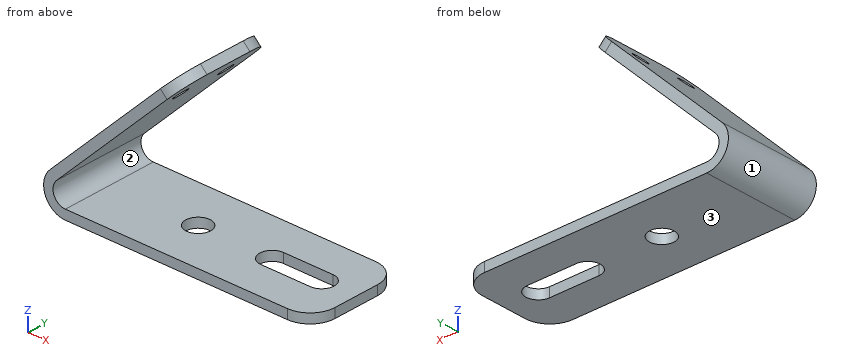
```python
from build123d import *

# Parameters (mm, degrees)
F1_DEPTH = 247.65
F2_R     = 38.1
F3_DEPTH = 50.8
F4_R     = 63.5
F5_DEPTH = 50.8
F6_R     = 127


with BuildPart() as f1:
    # F0 (on Front) → F1 (new body, symmetric)
    with BuildSketch(Plane.XZ):
        with BuildLine():
            Line((578.707208, 736.759715), (-79.026254, 79.026254))
            ThreePointArc((-79.026254, 79.026254), (-103.252777, -42.7687), (0, -111.76))
            Line((0, -111.76), (1270, -111.76))
            Line((1270, -111.76), (1270, -63.5))
            Line((1270, -63.5), (0, -63.5))
            ThreePointArc((0, -63.5), (-58.66635, -24.300398), (-44.901281, 44.901281))
            Line((-44.901281, 44.901281), (612.832181, 702.634742))
            Line((612.832181, 702.634742), (578.707208, 736.759715))
        make_face()
    extrude(amount=F1_DEPTH, both=True)

    # F2 (on face) → F3 (cut)
    with BuildSketch(Plane(origin=(-79.026254, 0, 79.026254), x_dir=(0, -1, 0), z_dir=(-0.707107, 0, 0.707107))):
        with Locations((-133.35, 739.675582)):
            Circle(F2_R)
        with Locations((121.92, 739.675582)):
            Circle(F2_R)
    extrude(amount=-F3_DEPTH, mode=Mode.SUBTRACT)

    # F4 (on face) → F5 (cut)
    with BuildSketch(Plane(origin=(0, 0, -111.76), x_dir=(1, 0, 0), z_dir=(0, 0, -1))):
        with BuildLine():
            Line((838.2, -63.5), (1092.2, -63.5))
            ThreePointArc((1092.2, -63.5), (1155.7, 0), (1092.2, 63.5))
            Line((1092.2, 63.5), (838.2, 63.5))
            ThreePointArc((838.2, 63.5), (774.7, 0), (838.2, -63.5))
        make_face()
        with Locations((457.2, 0)):
            Circle(F4_R)
    extrude(amount=-F5_DEPTH, mode=Mode.SUBTRACT)

    # F6
    f6_edges = [f1.edges().sort_by_distance(p)[0] for p in [
        (1270, -247.65, -87.63),
        (1270, 247.65, -87.63),
        (595.769694, -247.65, 719.697229),
        (595.769694, 247.65, 719.697229),
    ]]
    fillet(f6_edges, radius=F6_R)


solid = f1.part
```
Read the model definition and answer for the solid it produces. Units are mm, in the model's axes. Face numbers are marked on the shaded views. Give positions to 0.01 mm unless a question says otherwise; leave off trailing zeros. Order: outer loops, then holes, each group sorted by start corner. A loop starts at its lowest first (then second) coordinate and runs counter-clockwise, first axis right, second up.
(1) Find section A-A (y = 0). Give the vertices of the cut face in (x, z).
(2) Straight lines are drawn through the part: L1, parallel to X at y = 0, z = -92; L2, parallel to Y at x = 457, z = -84. For each, find the intervals that lie inside material, in ascending order.
(3) Find section B-B (x = 1000.5). Give the vertices of the cut face in (y, z).
(4) For a pull along Z with two mould halves and no side action, classify the marked faces 1, 2 and 3 as released by +Z, released by -Z, zero draft, split by the parting line, or undercut.
(5) Given pin 1 (1 mm diameter, centred on y = -159.5, z = 319, fed in from -X); pin 2 (12 mm diameter, centred on y = -85.5, z = 87, fed in from -X); pin 3 (1 mm diameter, centred on x = 232, y = 165, fed in from +Z), each flat-ended and moving along its own axis, determine where each tip first touches the part or whether it passes through.
(6) Find section D-D (y = -181.5). Give the vertices of the cut face in (x, z).
(7) Find section C-C (x = 808). Give the vertices of the cut face in (y, z).
Result sheet:
1. outline: (-79.03, 79.03) arc R111.76 ccw to (0, -111.76) - (393.7, -111.76) - (393.7, -63.5) - (0, -63.5) arc R63.5 cw to (-44.9, 44.9) - (612.83, 702.63) - (578.71, 736.76) - close; (520.7, -111.76) - (774.7, -111.76) - (774.7, -63.5) - (520.7, -63.5) - close; (1155.7, -111.76) - (1270, -111.76) - (1270, -63.5) - (1155.7, -63.5) - close
2. L1: x = -63.45 to 393.7, 520.7 to 774.7, 1155.7 to 1270
2. L2: y = -247.65 to -63.5, 63.5 to 247.65
3. outline: (-247.65, -111.76) - (-63.5, -111.76) - (-63.5, -63.5) - (-247.65, -63.5) - close; (63.5, -111.76) - (247.65, -111.76) - (247.65, -63.5) - (63.5, -63.5) - close
4. face 1: split by the parting line
4. face 2: undercut
4. face 3: released by -Z
5. pin 1: stops at x = 160.45
5. pin 2: stops at x = -77.05
5. pin 3: stops at z = 390.55
6. outline: (-79.03, 79.03) arc R111.76 ccw to (0, -111.76) - (1254.47, -111.76) - (1254.47, -63.5) - (0, -63.5) arc R63.5 cw to (-44.9, 44.9) - (601.85, 691.66) - (567.73, 725.78) - close
7. outline: (-247.65, -111.76) - (-55.86, -111.76) - (-55.86, -63.5) - (-247.65, -63.5) - close; (55.86, -111.76) - (247.65, -111.76) - (247.65, -63.5) - (55.86, -63.5) - close
